from build123d import *


with BuildPart() as part:
    # Sketch1 → Revolve1 (revolve)
    with BuildSketch(Plane.XY):
        with BuildLine():
            Line((-51.1302, 0), (-51.1302, -128.764609009))
            Line((-51.1302, -128.764609009), (-48.5902, -128.764609009))
            Line((-48.5902, -128.764609009), (-48.5902, -132.066609009))
            Line((-48.5902, -132.066609009), (-51.1302, -132.066609009))
            Line((-51.1302, -132.066609009), (-51.1302, -138.416609009))
            Line((-51.1302, -138.416609009), (-48.5902, -138.416609009))
            Line((-48.5902, -138.416609009), (-48.5902, -141.718609009))
            Line((-48.5902, -141.718609009), (-51.1302, -141.718609009))
            Line((-51.1302, -141.718609009), (-51.1302, -148.068609009))
            Line((-51.1302, -148.068609009), (-44.45, -148.068609009))
            Line((-44.45, -148.068609009), (-16.477563907, -43.674056299))
            ThreePointArc((-16.477563907, -43.674056299), (-16.311628933, -42.839844852), (-16.256, -41.99111134))
            ThreePointArc((-16.256, -41.99111134), (-17.493414319, -35.770209463), (-21.017272165, -30.496383505))
            Line((-21.017272165, -30.496383505), (-40.018927835, -11.494727835))
            ThreePointArc((-40.018927835, -11.494727835), (-43.542785681, -6.220901877), (-44.7802, 0))
            Line((-44.7802, 0), (-51.1302, 0))
        make_face()
    revolve(axis=Axis((0, 0, 0), (0, -1, 0)))


solid = part.part
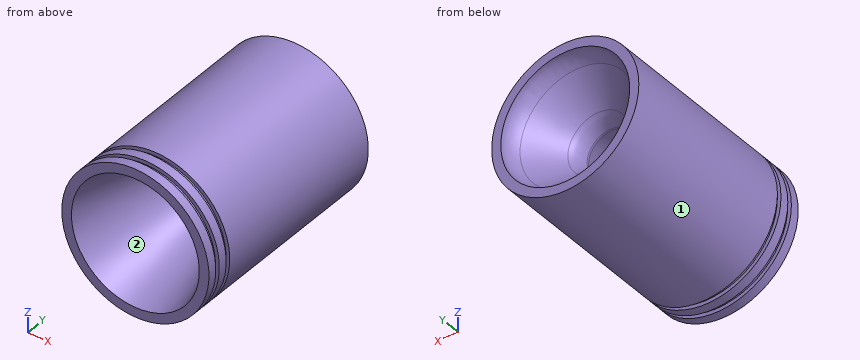
The listing builds one solid part. Answer for the finished solid, in the listing's coordinates (mm). Face numbers are marked on the shaded views. Give positions to 0.01 mm unless a question says otherwise; leave off trailing zeros. Loops run counter-clockwise (first coordinate to the right, second up) from the corner with the lowest first, then second, coordinate; pieces in that order, holes last.
Item 1: Determine the mould class of the marked faces 1 and 2 for opening direction Z: +Z half, -Z half, draft (parallel to the pull), parting line (faces both ways), or undercut.
Derived:
face 1: parting line
face 2: undercut
Item 2: A cutting plane is placed at C-C (y = -66.5). Give the vertices of the cut face in (x, z), then the cut area to 3 significant figures.
Derived:
outline: circle Ø102.26 at (0, 0); hole circle Ø45.19 at (0, 0)
area: 6,610 mm2
Item 3: A cutting plane is placed at D-D (y = -105.5). Give the vertices of the cut face in (x, z).
Derived:
outline: circle Ø102.26 at (0, 0); hole circle Ø66.09 at (0, 0)
Item 4: Each of these flat-tipped pins is pushed along its axis until it touches: pin 1 Ø12 at (y, z) = (-85.5, -30) entering from -X; pin 2 Ø8 at (x, y) = (-34.5, -35.5) entering from +Z; pin 3 Ø1.5 at (y, z) = (-118.5, -18) entering from -X. Where does it stop, or does it pass through?
Derived:
pin 1: stops at x = -45.15
pin 2: stops at z = 41.04
pin 3: stops at x = -48.13
Item 5: Find the intervals of material crossed by line 1 along Z through (x, y) = (0, -39); line 2 along X through (y, z) = (-74, 19); line 3 along Z through (x, y) = (33.5, -125.5), in increasing order.
Derived:
line 1: z = -51.13 to -16.53, 16.53 to 51.13
line 2: x = -47.47 to -15.63, 15.63 to 47.47
line 3: z = -38.63 to -18.78, 18.78 to 38.63
